Geometry: final body of the model. Coordinates: model frame, mm. A direction names the side the tool comes from. Coordinates: 2 decimals unless noted, no trailing zeros. Write each loop counter-clockwise with the first axis right and the second up, starting at its lowest first coordinate (ties: lowest second). Pieces come first, ordered by that corner, then holes.
from build123d import *

# Parameters (mm, degrees)
SKETCH1_W           = 381
SKETCH1_H           = 44.45
SKETCH1_R           = 9.525
BOSS_EXTRUDE1_DEPTH = 6.35
FILLET1_R           = 5.08
SKETCH2_W           = 50.8
SKETCH2_H           = 6.35
CUT_EXTRUDE1_DEPTH  = 7.35


with BuildPart() as part:
    # Sketch1 → Boss-Extrude1 (new body)
    with BuildSketch(Plane.XY):
        with Locations((1295.4, -50.8)):
            Rectangle(SKETCH1_W, SKETCH1_H)
        with Locations((1219.2, -50.8)):
            Circle(SKETCH1_R, mode=Mode.SUBTRACT)
        with Locations((1397, -50.8)):
            Circle(SKETCH1_R, mode=Mode.SUBTRACT)
    extrude(amount=BOSS_EXTRUDE1_DEPTH)

    # Fillet1
    fillet1_edges = [part.edges().sort_by_distance(p)[0] for p in [
        (1104.9, -28.575, 3.175),
        (1485.9, -28.575, 3.175),
        (1485.9, -73.025, 3.175),
        (1104.9, -73.025, 3.175),
    ]]
    fillet(fillet1_edges, radius=FILLET1_R)

    # Sketch2 → Cut-Extrude1 (cut, through all)
    with BuildSketch(Plane.XY.offset(6.35)):
        with Locations((1331.11875, -44.45)):
            Rectangle(SKETCH2_W, SKETCH2_H)
    extrude(amount=-CUT_EXTRUDE1_DEPTH, mode=Mode.SUBTRACT)


solid = part.part
Item 1: Pull-direction query (Y, two-part tool) for faces 3 (the flat face through (1104.9, -51, 3)), 4 (the cylindrical face through (1406.085, -47.939, 3.131)), 5 (the flat face through (1293, -28.575, 3)); classes: released by +Y, released by -Y, zero draft, split by the parting line, or undercut.
Derived:
face 3: zero draft
face 4: undercut
face 5: released by +Y
Item 2: Section A-A, the plane y = -50.8. Output: boundary loops of the cut face in (x, z) (3 decimals), plus the area to 3 significant figures.
Derived:
outline: (1104.9, 0) - (1209.675, 0) - (1209.675, 6.35) - (1104.9, 6.35) - close; (1228.725, 0) - (1387.475, 0) - (1387.475, 6.35) - (1228.725, 6.35) - close; (1406.525, 0) - (1485.9, 0) - (1485.9, 6.35) - (1406.525, 6.35) - close
area: 2,180 mm2
Item 3: Section D-D, the plane x = 1402. Output: boundary loops of the cut face in (y, z) (3 decimals), plus the area to 3 significant figures.
Derived:
outline: (-73.025, 0) - (-58.907, 0) - (-58.907, 6.35) - (-73.025, 6.35) - close; (-42.693, 0) - (-28.575, 0) - (-28.575, 6.35) - (-42.693, 6.35) - close
area: 179 mm2
Item 4: Set-up query: faces 1 (the flat face through (1356.519, -44, 3)), 2 (the flat face through (1293, -50, 6.35)). Return all of +Z, -Z, +X, -X, +Y, -Y with unobstructed straight access to the full face (end or side cutting, diameter ignored); none if empty.
Derived:
face 1: +Z, -Z
face 2: +Z, +X, -X, +Y, -Y
Item 5: Material intervals for probe 1 along Y at (x, z) = (1334, 3.5) (3 decimals); probe 2 along Y at (x, z) = (1397, 2.25) (3 decimals); probe 3 along X at (y, z) = (-45.5, 1.75), sorted ascending.
Derived:
probe 1: y = -73.025 to -47.625, -41.275 to -28.575
probe 2: y = -73.025 to -60.325, -41.275 to -28.575
probe 3: x = 1104.9 to 1211.29, 1227.11 to 1305.72, 1356.52 to 1389.09, 1404.91 to 1485.9
Item 6: Section C-C, the plane z = 4.75. Output: boundary loops of the cut face in (x, y) (3 decimals), plus the area to 3 significant figures.
Derived:
outline: (1104.9, -67.945) arc R5.08 ccw to (1109.98, -73.025) - (1480.82, -73.025) arc R5.08 ccw to (1485.9, -67.945) - (1485.9, -33.655) arc R5.08 ccw to (1480.82, -28.575) - (1109.98, -28.575) arc R5.08 ccw to (1104.9, -33.655) - close; hole circle Ø19.05 at (1219.2, -50.8); hole (1305.719, -47.625) - (1356.519, -47.625) - (1356.519, -41.275) - (1305.719, -41.275) - close; hole circle Ø19.05 at (1397, -50.8)
area: 16,000 mm2
Item 7: Section B-B, the plane x = 1219.2. Output: boundary loops of the cut face in (y, z) (3 decimals).
Derived:
outline: (-73.025, 0) - (-60.325, 0) - (-60.325, 6.35) - (-73.025, 6.35) - close; (-41.275, 0) - (-28.575, 0) - (-28.575, 6.35) - (-41.275, 6.35) - close
